```python
from build123d import *

# Parameters (mm, degrees)
SKETCH_1_W          = 30
SKETCH_1_H          = 180
EXTRUDE_1_DEPTH     = 12
SKETCH_2_R          = 5.5
CUT_EXTRUDE_1_DEPTH = 12
CHAMFER_1_SIZE      = 6


with BuildPart() as part:
    # 草图1 → 凸台-拉伸1 (new body)
    with BuildSketch(Plane.XY):
        Rectangle(SKETCH_1_W, SKETCH_1_H)
    extrude(amount=EXTRUDE_1_DEPTH)

    # 草图2 → 切除-拉伸1 (cut)
    with BuildSketch(Plane.XY.offset(12)):
        with Locations((0, -75)):
            Circle(SKETCH_2_R)
        with BuildLine():
            Line((4.5, 35), (4.5, -55))
            ThreePointArc((4.5, -55), (0, -59.5), (-4.5, -55))
            Line((-4.5, -55), (-4.5, 35))
            ThreePointArc((-4.5, 35), (0, 39.5), (4.5, 35))
        make_face()
    extrude(amount=-CUT_EXTRUDE_1_DEPTH, mode=Mode.SUBTRACT)

    # 倒角1
    chamfer_1_edges = [part.edges().sort_by_distance(p)[0] for p in [
        (15, 90, 6),
    ]]
    chamfer(chamfer_1_edges, length=CHAMFER_1_SIZE)


solid = part.part
```
CAD build for the part. Positions are in the model's coordinates, mm. A direction names the side the tool comes from. Give positions to 0.01 mm unless a question says otherwise; leave off trailing zeros. Write each loop counter-clockwise with the first axis right and the second up, starting at its lowest first coordinate (ties: lowest second). Pieces come first, ordered by that corner, then holes. Notation, with made-up numbers: M 68,82 L 77,82 A24 ccw 77,116 Z; hole C 39,28 d4. An arc over 180 degrees is marked long. Return JSON: item names as keys, results as strings. Group by question number.
(1) 3-axis set-ups, long thin cutter, end or side, ignore diameter. For faces 4 (the face through (-3, 90, 6)), 5 (the face through (-0.1, 39.5, 6.1)): which of +Z, -Z, +X, -X, +Y, -Y reach the whole face in a straight line?
(2) Band-saw the part on B-B (y = -75). Give the cut face in (x, z), and give its area (3 significant figures).
(3) Band-saw the part on C-C (z = 3). Give the cut face in (x, y), and give its area (3 significant figures).
(4) Band-saw the part on A-A (x = 0). Give the cut face in (y, z), and give its area (3 significant figures).
(5) Mould opens along X. For faces 1 (the face through (-7, 1, 12)), 2 (the face through (15, -4, 6)), 3 (the face through (-0.716, -69.547, 6.084)) say: pulls with the +X half, pulls with the -X half, needs draft (parallel to the pull), parting line crosses it, or undercut.
(6) Flat gauge pins, fed straight in: pin 1 Ø1.5 at (x, y) = (7, -67.5) entering from -Z; pin 2 Ø9 at (x, y) = (0, -75) entering from -Z. Where does each tip first touch, or does it go through?
(7) Drill centre lines: L1, parallel to Y at x = 0, z = 6.5; L2, parallel to X at y = -22, z = 8; L3, parallel to Y at x = 3.5, z = 7.75. Where is each one in solid material? Low to high. Write a range as [from, to].
Entries:
{
 "1": {"face 4": "+Z, -Z, +X, -X, +Y", "face 5": "+Z, -Z"},
 "2": {"outline": "M -15,0 L -5.5,0 L -5.5,12 L -15,12 Z; M 5.5,0 L 15,0 L 15,12 L 5.5,12 Z", "area": "228 mm^2"},
 "3": {"outline": "M -15,-90 L 15,-90 L 15,84 L 9,90 L -15,90 Z; hole C 0,-75 d11; hole M -4.5,-55 A4.5 ccw 4.5,-55 L 4.5,35 A4.5 ccw -4.5,35 Z", "area": "4,410 mm^2"},
 "4": {"outline": "M -90,0 L -80.5,0 L -80.5,12 L -90,12 Z; M -69.5,0 L -59.5,0 L -59.5,12 L -69.5,12 Z; M 39.5,0 L 90,0 L 90,12 L 39.5,12 Z", "area": "840 mm^2"},
 "5": {"face 1": "needs draft", "face 2": "pulls with the +X half", "face 3": "undercut"},
 "6": {"pin 1": "stops at z = 0", "pin 2": "passes through"},
 "7": {"L1": "y = [-90, -80.5], [-69.5, -59.5], [39.5, 90]", "L2": "x = [-15, -4.5], [4.5, 15]", "L3": "y = [-90, -79.24], [-70.76, -57.83], [37.83, 90]"}
}
